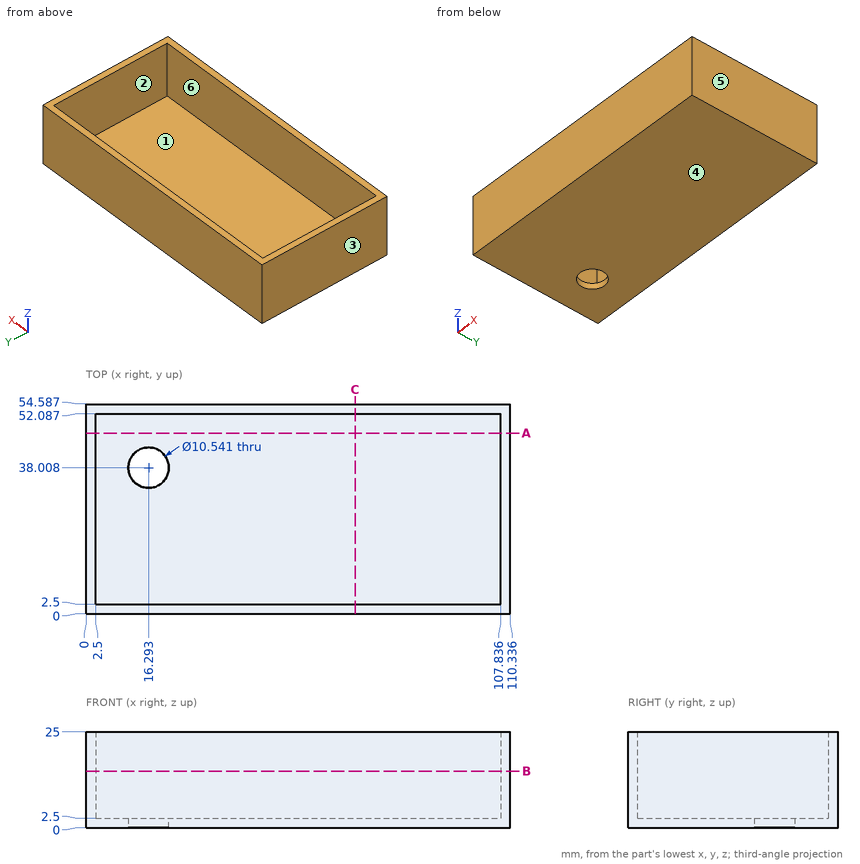
Source: three-view drawing plus pictorial views. Frame: mm from the lowest corner of the part. A direction names the side the tool comes from. Give positions to 0.01 mm unless a question says otherwise; leave off trailing zeros. Order: outer loops, then holes, each group sorted by start corner. A loop starts at its lowest first (then second) coordinate and runs counter-clockwise, first axis right, second up.
1. Section C-C on x = 70. Return the cut outline in (y, z).
Derived:
outline: (0, 0) - (54.59, 0) - (54.59, 25) - (52.09, 25) - (52.09, 2.5) - (2.5, 2.5) - (2.5, 25) - (0, 25) - close
2. Section B-B on z = 14.75. Return the cut outline in (x, y) (1 decimal).
Derived:
outline: (0, 0) - (110.3, 0) - (110.3, 54.6) - (0, 54.6) - close; hole (2.5, 2.5) - (107.8, 2.5) - (107.8, 52.1) - (2.5, 52.1) - close
3. Section A-A on y = 47. Return the cut outline in (x, z) (1 decimal).
Derived:
outline: (0, 0) - (110.3, 0) - (110.3, 25) - (107.8, 25) - (107.8, 2.5) - (2.5, 2.5) - (2.5, 25) - (0, 25) - close
4. Pin query (flat end, axial travel): pin 1 (11 mm diameter, centred on x = 60.5, z = 16, fed in from -Y); pin 2 (12 mm diameter, centred on x = 44, y = 29.5, fed in from +Z); pin 3 (9.5 mm diameter, centred on x = 16.29, y = 38.01, fed in from +Z). Return the tip coordinate at first contact, or that it passes through.
Derived:
pin 1: stops at y = 0
pin 2: stops at z = 2.5
pin 3: passes through
5. Material intervals for L1, parallel to Y at x = 32.5, z = 7.75; L2, parallel to X at y = 27, z = 19.75 (1 decimal); L3, parallel to Z at x = 47, y = 10.5, sorted ascending.
Derived:
L1: y = 0 to 2.5, 52.09 to 54.59
L2: x = 0 to 2.5, 107.8 to 110.3
L3: z = 0 to 2.5
6. Reachability of the marked faces 5 and 6 from +Z, -Z, +X, -X, +Y, -Y: full face, straight path, thin tool, end or side. Return the list, or none.
Derived:
face 5: +Z, -Z, +X, +Y, -Y
face 6: +Z
7. Mould query, pull axis X, two halves, no side actions, for the marked faces 1, 2, 3 and 4. Classes: released by +X, released by -X, zero draft, split by the parting line, or undercut.
Derived:
face 1: undercut
face 2: undercut
face 3: released by -X
face 4: zero draft
